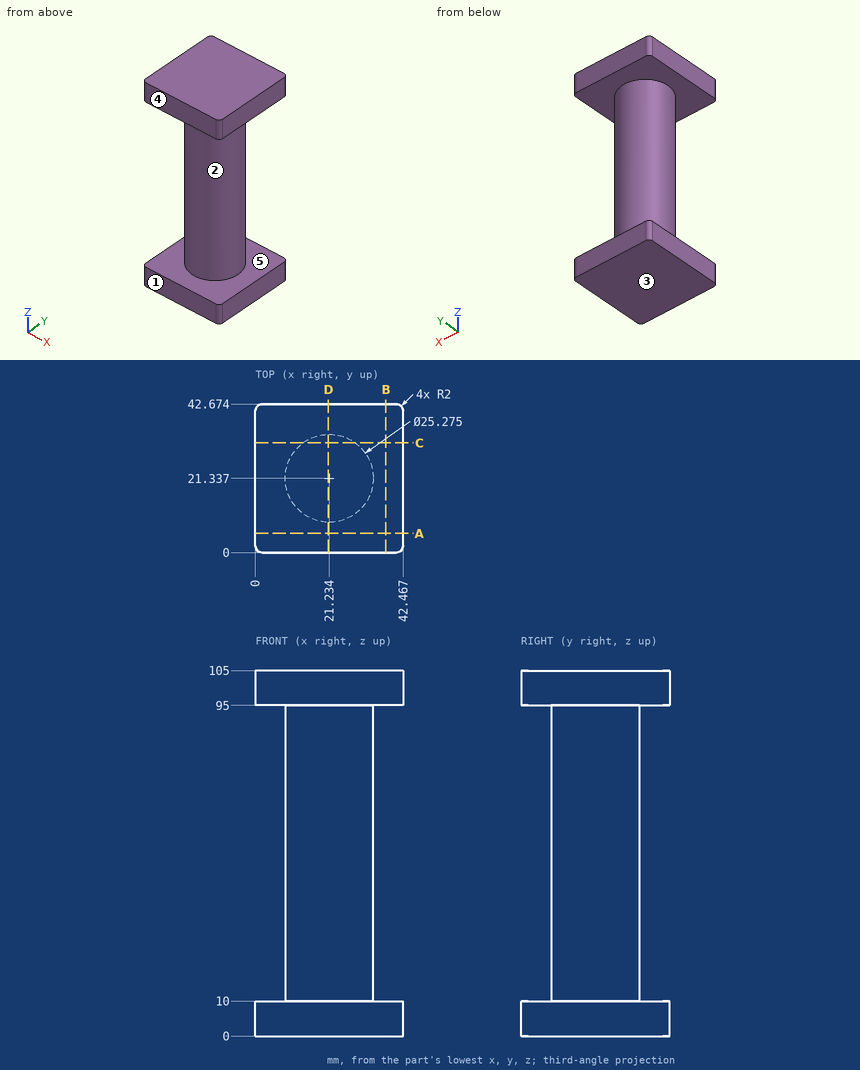
Could you check a few things on this drawing? It's one solid part, dimensions in mm from its lowest x, y, z. A direction names the side the tool comes from. Coordinates: 2 decimals unless noted, no trailing zeros. Order: outer loops, then holes, each group sorted by start corner. A loop starts at its lowest first (then second) coordinate and runs counter-clockwise, first axis right, second up. Notation, with made-up numbers: M 1.5,52 L 27.5,52 A22 ccw 27.5,74 Z; hole C 65,32.5 d7. An arc over 180 degrees is marked long. Use a Markdown table: item, result. Add a question column.
Q1. Which directions (+Z, -Z, +X, -X, +Y, -Y) give clear straight access to the entire face, cutting with the end or side of a thin tool? Please do the marked faces 1 and 2.
Q2. I want a section at B-B on x = 37.5. List the corners of the cut face in (y, z) for me (1 decimal).
Q3. I want a section at A-A on y = 5.5. List the corners of the cut face in (x, z) for me.
Q4. We'd pull the mould along Z, two halves only. Please class the marked faces 3, 4 and 5: pulls with the +Z half, pulls with the -Z half, needs draft (parallel to the pull), parting line crosses it, or undercut.
Q5. I'm going to push a flat-ended pin straight in: pin 1 (5 mm diameter, centred on x = 24.5, z = 65.5, fed in from +Y). Where does the tip first touch, or does it pass through?
Q6. I want a section at C-C on y = 31.5. List the corners of the cut face in (x, z) for me (1 decimal), then the cut area to 3 significant figures.
Q7. I want a section at D-D on x = 21. List the corners of the cut face in (y, z) for me (1 decimal), then the cut area to 3 significant figures.
Q8. If I drill on L1, parallel to Z at x = 7.5, y = 22.5; L2, parallel to X at y = 22, z = 10.5; L3, parallel to Y at x = 21, z = 83, over which ranges is the centre line in solid material (lowest first)?
Checked values:
| question | item | result |
|---|---|---|
| 1 | face 1 | +Z, -Z, +X, -X, -Y |
| 1 | face 2 | none |
| 2 | outline | M 0,0 L 42.7,0 L 42.7,10 L 0,10 Z; M 0,95 L 42.7,95 L 42.7,105 L 0,105 Z |
| 3 | outline | M 0,0 L 42.47,0 L 42.47,10 L 0,10 Z; M 0,95 L 42.47,95 L 42.47,105 L 0,105 Z |
| 4 | face 3 | pulls with the -Z half |
| 4 | face 4 | needs draft |
| 4 | face 5 | undercut |
| 5 | pin 1 | y = 33.95 |
| 6 | outline | M 0,0 L 42.5,0 L 42.5,10 L 28.7,10 L 28.7,95 L 42.5,95 L 42.5,105 L 0,105 L 0,95 L 13.7,95 L 13.7,10 L 0,10 Z |
| 6 | area | 2,130 mm² |
| 7 | outline | M 0,0 L 42.7,0 L 42.7,10 L 34,10 L 34,95 L 42.7,95 L 42.7,105 L 0,105 L 0,95 L 8.7,95 L 8.7,10 L 0,10 Z |
| 7 | area | 3,000 mm² |
| 8 | L1 | 0 to 10, 95 to 105 |
| 8 | L2 | 8.61 to 33.85 |
| 8 | L3 | 8.7 to 33.97 |
